```python
from build123d import *

# Parameters (mm, degrees)
SKETCH3_W              = 914.4
SKETCH3_H              = 609.6
BOSS_EXTRUDE1_DEPTH    = 0.79375
SKETCH4_OUTSIDE_W      = 1136.194
SKETCH4_OUTSIDE_H      = 831.394
CUT_EXTRUDE1_DEPTH     = 2.54
F_4_CLEARANCE_HOLE1_D  = 3.2639
F_10_CLEARANCE_HOLE1_D = 5.1054


with BuildPart() as part:
    # Sketch3 → Boss-Extrude1 (new, symmetric)
    with BuildSketch(Plane.XY):
        Rectangle(SKETCH3_W, SKETCH3_H)
    extrude(amount=BOSS_EXTRUDE1_DEPTH, both=True)

    # Sketch4 outside → Cut-Extrude1 (cut)
    with BuildSketch(Plane(origin=(0, 0, -0.79375), x_dir=(-1, 0, 0), z_dir=(0, 0, -1))):
        Rectangle(SKETCH4_OUTSIDE_W, SKETCH4_OUTSIDE_H)
        Polygon((387.349825772, -19.107241188), (212.724825222, -19.107241187), (212.724825222, 123.767758813), (387.349825755, 123.767758812), align=None, mode=Mode.SUBTRACT)
    extrude(amount=-CUT_EXTRUDE1_DEPTH, mode=Mode.SUBTRACT)

    # #4 Clearance Hole1 (through all)
    with Locations(Plane(origin=(0, 0, -0.79375), x_dir=(-1, 0, 0), z_dir=(0, 0, -1))):
        with Locations((350.837325504, 115.830258819), (249.237325504, 115.830258806), (249.23732552, -11.169741194), (350.83732552, -11.169741181)):
            Hole(F_4_CLEARANCE_HOLE1_D / 2)

    # #10 Clearance Hole1 (through all)
    with Locations(Plane(origin=(0, 0, -0.79375), x_dir=(-1, 0, 0), z_dir=(0, 0, -1))):
        with Locations((220.027325222, 1.530258305), (220.027325222, 103.129958819), (380.047325758, 103.130259319), (380.04732577, 1.530558805)):
            Hole(F_10_CLEARANCE_HOLE1_D / 2)


solid = part.part
```
Read the model definition and answer for the solid it produces. Units are mm, in the model's axes. Give positions to 0.01 mm unless a question says otherwise; leave off trailing zeros.
(1) Straight lines are drawn through the part: L1, parallel to Y at x = -220, z = 0.6; L2, parallel to X at y = 103.5, z = -0.2. For each, find the intervals that lie inside material, in ascending order.
(2) For a pull along Y with two mould halves and no side action, classify faces 1 (the cylindrical face through (-382.6, 103.2, 0)), 2 (the flat face through (-301, 53, 0.794)) as released by +Y, released by -Y, zero draft, split by the parting line, or undercut.
(3) Given pin 1 (2 mm diameter, centred on x = -350.84, y = -11.17, fed in from +Z), flat-ended and moving along its own axis, determine where the tip first touches the part or whether it passes through.
Result sheet:
1. L1: y = -19.11 to -1.02, 4.08 to 100.58, 105.68 to 123.77
1. L2: x = -387.35 to -382.57, -377.52 to -222.55, -217.5 to -212.72
2. face 1: undercut
2. face 2: zero draft
3. pin 1: passes through
